Work out the finished part from the listing and answer in its coordinate system (mm). Face numbers are marked on the shaded views. A direction names the side the tool comes from. Give positions to 0.01 mm unless a question says otherwise; leave off trailing zeros. Order: outer loops, then holes, each group sorted by start corner. A loop starts at its lowest first (then second) coordinate and runs counter-clockwise, first axis right, second up. Notation, with made-up numbers: M 22,-26 L 53,-26 A33 cw 53,3 Z; hole C -6,40.5 d1. An arc over 180 degrees is marked long. One line per item, written item: value.
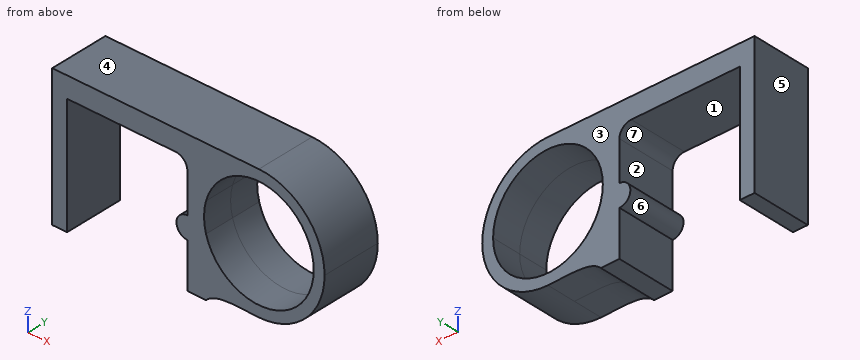
from build123d import *

# Parameters (mm, degrees)
F1_DEPTH = 5


with BuildPart() as f1:
    # F0 (on Front) → F1 (new body, symmetric)
    with BuildSketch(Plane.XZ):
        with BuildLine():
            Line((-24.5694083333, 31.5104130507), (-50.5694083333, 31.5104130507))
            Line((-50.5694083333, 31.5104130507), (-50.5694083333, 8.0104130507))
            Line((-50.5694083333, 8.0104130507), (-48.0694083333, 8.0104130507))
            Line((-48.0694083333, 8.0104130507), (-48.0694083333, 28.0104130507))
            Line((-48.0694083333, 28.0104130507), (-29.7194083333, 28.0104130507))
            ThreePointArc((-29.7194083333, 28.0104130507), (-28.3051947709, 27.424626613), (-27.7194083333, 26.0104130507))
            Line((-27.7194083333, 26.0104130507), (-27.7194083333, 19.3554483443))
            Line((-27.7194083333, 19.3554483443), (-27.7194083333, 15.665377757))
            Line((-27.7194083333, 15.665377757), (-27.7194083333, 8.0104130507))
            Line((-27.7194083333, 8.0104130507), (-24.5694083333, 8.0104130507))
            Line((-24.5694083333, 8.0104130507), (-24.5694083333, 13.8020069146))
            ThreePointArc((-24.5694083333, 13.8020069146), (-26.7411284149, 20.4004295021), (-24.5694083333, 26.9988520897))
            Line((-24.5694083333, 26.9988520897), (-24.5694083333, 31.5104130507))
        make_face()
        with BuildLine():
            ThreePointArc((-15.6311448663, 31.5104130507), (-20.6373094688, 30.3185971969), (-24.5694083333, 26.9988520897))
            Line((-24.5694083333, 26.9988520897), (-24.5694083333, 22.8769333271))
            ThreePointArc((-24.5694083333, 22.8769333271), (-14.3814986476, 29.5908598146), (-6.3561448663, 20.4004295021))
            ThreePointArc((-6.3561448663, 20.4004295021), (-14.3814986476, 11.2099991897), (-24.5694083333, 17.9239256771))
            Line((-24.5694083333, 17.9239256771), (-24.5694083333, 13.8020069146))
            ThreePointArc((-24.5694083333, 13.8020069146), (-20.6371443338, 10.4821784577), (-15.630774911, 9.2904459598))
            ThreePointArc((-15.630774911, 9.2904459598), (-7.7750693624, 12.5446155962), (-4.5211613178, 20.4004295021))
            ThreePointArc((-4.5211613178, 20.4004295021), (-7.7752001603, 28.2563742082), (-15.6311448663, 31.5104130507))
        make_face()
        with BuildLine():
            Line((-24.5694083333, 22.8769333271), (-24.5694083333, 26.9988520897))
            ThreePointArc((-24.5694083333, 26.9988520897), (-26.7411284149, 20.4004295021), (-24.5694083333, 13.8020069146))
            Line((-24.5694083333, 13.8020069146), (-24.5694083333, 17.9239256771))
            ThreePointArc((-24.5694083333, 17.9239256771), (-24.9061448663, 20.4004295021), (-24.5694083333, 22.8769333271))
        make_face()
        with BuildLine():
            ThreePointArc((-15.630774911, 9.2904459598), (-20.6371443338, 10.4821784577), (-24.5694083333, 13.8020069146))
            Line((-24.5694083333, 13.8020069146), (-24.5694083333, 8.0104130507))
            add(Edge.make_bspline(
                [(-24.5694083333, 8.0104130507), (-22.6878308277, 9.9391806871), (-18.7427580517, 9.2241163725), (-15.630774911, 9.2904459598)],
                knots=[0, 0, 0, 0, 9.029820137, 9.029820137, 9.029820137, 9.029820137], degree=3))
        make_face()
        with BuildLine():
            Line((-27.7194083333, 15.665377757), (-27.7194083333, 19.3554483443))
            ThreePointArc((-27.7194083333, 19.3554483443), (-29.564443627, 17.5104130507), (-27.7194083333, 15.665377757))
        make_face()
        with BuildLine():
            Line((-15.6311448663, 31.5104130507), (-24.5694083333, 31.5104130507))
            Line((-24.5694083333, 31.5104130507), (-24.5694083333, 26.9988520897))
            ThreePointArc((-24.5694083333, 26.9988520897), (-20.6373094688, 30.3185971969), (-15.6311448663, 31.5104130507))
        make_face()
    extrude(amount=F1_DEPTH, both=True)


solid = f1.part
(1) Section B-B, the plane x = -12.5 is taken. Give the vertices of the cut face in (y, z).
Findings:
outline: M -5,9.74 L 5,9.74 L 5,11.67 L -5,11.67 Z; M -5,29.13 L 5,29.13 L 5,31.06 L -5,31.06 Z
(2) Find the intervals of material crossed by probe 1 along X at (y, z) = (-2.5, 20.5); probe 2 along X at (y, z) = (-0.5, 12); probe 3 along Z at (x, y) = (-48, 1.75), in increasing order. Write a range as from..to.
Findings:
probe 1: x = -50.57..-48.07, -27.72..-24.91, -6.36..-4.52
probe 2: x = -50.57..-48.07, -27.72..-19.56, -11.7..-8.36
probe 3: z = 28.01..31.51
(3) Given P1, Ø6, axis at x = -36, z = 23.5, coming from the -Y side; P2, Ø4, axis at y = -1, z = 27.5, coming from the +X side; P3, Ø6, axis at y = 0.5, z = 26, coming from the +X side, each flat-ended and moving along its own axis, determine where each tip first touches the part or whether it passes through.
Findings:
P1: passes through
P2: stops at x = -5.76
P3: stops at x = -4.83
(4) Section D-D, the plane x = -29 is taken. Give the vertices of the cut face in (y, z).
Findings:
outline: M -5,16.18 L 5,16.18 L 5,18.84 L -5,18.84 Z; M -5,27.88 L 5,27.88 L 5,31.51 L -5,31.51 Z
(5) Which of the six approach directions +Z, -Z, +X, -X, +Y, -Y give full straight-line access (tool end or side, diameter ignored) to the marked faces 1, 2 and 3?
Findings:
face 1: -Z, +Y, -Y
face 2: +Y, -Y
face 3: +Z, -Z, +X, -X, +Y
(6) Section A-A, the plane z = 17 is taken. Give the vertices of the cut face in (x, y).
Findings:
outline: M -50.57,-5 L -48.07,-5 L -48.07,5 L -50.57,5 Z; M -29.49,-5 L -24.26,-5 L -24.26,5 L -29.49,5 Z; M -7,-5 L -5.05,-5 L -5.05,5 L -7,5 Z
(7) Determine the mould class of the marked faces 4, 5, 6 and 7 for opening direction X: pulls with the +X half, pulls with the -X half, needs draft (parallel to the pull), parting line crosses it, or undercut.
Findings:
face 4: needs draft
face 5: pulls with the -X half
face 6: undercut
face 7: undercut
(8) Section C-C, the plane z = 13.25 is taken. Give the vertices of the cut face in (x, y), then the cut area to 3 significant figures.
Findings:
outline: M -50.57,-5 L -48.07,-5 L -48.07,5 L -50.57,5 Z; M -27.72,-5 L -21.54,-5 L -21.54,5 L -27.72,5 Z; M -9.72,-5 L -7.13,-5 L -7.13,5 L -9.72,5 Z
area: 113 mm^2
